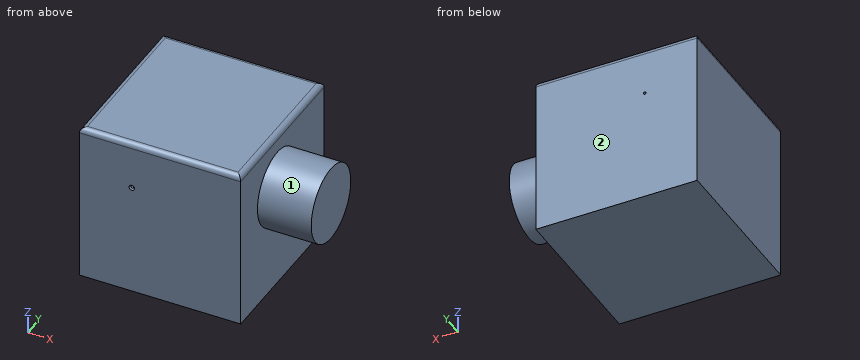
```python
from build123d import *

# Parameters (mm, degrees)
F0_W           = 381
F0_H           = 381
F1_DEPTH       = 381
F3_D           = 6.35
F3_CSINK_D     = 12.7
F3_CSINK_ANGLE = 90
F4_R           = 12.7
F5_R           = 90.072303
F6_DEPTH       = 127


with BuildPart() as f1:
    # F0 (on Front) → F1 (new body)
    with BuildSketch(Plane.XZ):
        with Locations((190.5, 190.5)):
            Rectangle(F0_W, F0_H)
    extrude(amount=F1_DEPTH)

    # F3 (through all)
    with Locations(Plane.XZ.offset(381)):
        with Locations((123.825006, 267.081022)):
            CounterSinkHole(F3_D / 2, F3_CSINK_D / 2, counter_sink_angle=F3_CSINK_ANGLE)

    # F4
    f4_edges = [f1.edges().sort_by_distance(p)[0] for p in [
        (381, -190.5, 381),
        (0, -190.5, 381),
        (190.5, 0, 381),
        (190.5, -381, 381),
    ]]
    fillet(f4_edges, radius=F4_R)

    # F5 (on face) → F6 (join)
    with BuildSketch(Plane.YZ.offset(381)):
        with Locations((-214.303002, 247.298166)):
            Circle(F5_R)
    extrude(amount=F6_DEPTH)


solid = f1.part
```
Input: part model. Units: mm. Frame: model coordinates. Face numbers are marked on the shaded views. A direction names the side the tool comes from. Coordinates: 2 decimals unless noted, no trailing zeros. Write each loop counter-clockwise with the first axis right and the second up, starting at its lowest first coordinate (ties: lowest second). Pieces come first, ordered by that corner, then holes.
1) Section B-B on y = -61.5. Output: boundary loops of the cut face in (x, z) (3 decimals), and give its area (3 significant figures).
2) Pin query (flat end, axial travel): pin 1 Ø10 at (x, z) = (123.83, 267.08) entering from -Y; pin 2 Ø12 at (y, z) = (-248, 156.5) entering from +X. Return the tip coordinate at first contact, or that it passes through.
3) Section D-D on z = 128. Output: boundary loops of the cut face in (x, y).
4) Set-up query: the marked faces 1 and 2. Return all of +Z, -Z, +X, -X, +Y, -Y with unobstructed straight access to the full face (end or side cutting, diameter ignored); none if empty.
5) Section A-A on z = 307. Output: boundary loops of the cut face in (x, y).
6) Section C-C on x = 407. Output: boundary loops of the cut face in (y, z), and give its area (3 significant figures).
7) Material intervals for line 1 along X through (y, z) = (-140, 337); line 2 along Z through (x, y) = (452, -220.5); line 3 along Z through (x, y) = (437.5, -221.5), sorted ascending.
Check result:
1. outline: (0, 0) - (381, 0) - (381, 368.3) arc R12.7 ccw to (368.3, 381) - (12.7, 381) arc R12.7 ccw to (0, 368.3) - close; hole circle Ø6.35 at (123.825, 267.081)
1. area: 145,000 mm2
2. pin 1: stops at y = -379.66
2. pin 2: stops at x = 381
3. outline: (0, -381) - (381, -381) - (381, 0) - (0, 0) - close
4. face 1: +X
4. face 2: +Z, -Z, +X, -X, +Y
5. outline: (0, -381) - (381, -381) - (381, -281.75) - (508, -281.75) - (508, -146.86) - (381, -146.86) - (381, 0) - (0, 0) - close
6. outline: circle Ø180.14 at (-214.3, 247.3)
6. area: 25,500 mm2
7. line 1: x = 0 to 381
7. line 2: z = 157.44 to 337.16
7. line 3: z = 157.51 to 337.08
